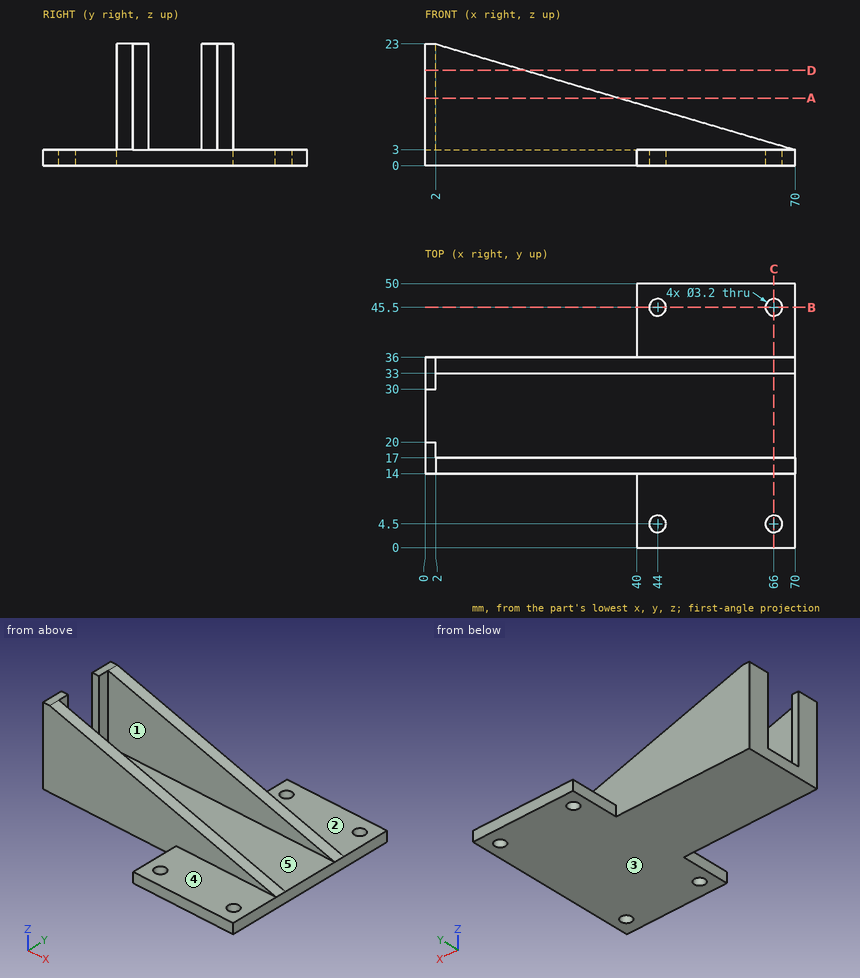
Input: dimensioned drawing with shaded views. Units: mm. Origin: part minimum x, y, z. A direction names the side the tool comes from. Coordinates: 2 decimals unless noted, no trailing zeros. Write each loop counter-clockwise with the first axis right and the second up, starting at its lowest first coordinate (ties: lowest second). Pieces come first, ordered by that corner, then holes. Notation, with made-up numbers: M 87,33.5 L 118,33.5 A24 cw 118,55.5 Z; hole C 87,83 d1. An arc over 180 degrees is marked long. Use one line per item in the form item = value.
Q1. Section D-D (z = 18). Return loops of the section in (x, y), plus the area to 3 significant figures.
Answer below:
outline = M 0,14 L 19,14 L 19,17 L 2,17 L 2,20 L 0,20 Z; M 0,30 L 2,30 L 2,33 L 19,33 L 19,36 L 0,36 Z
area = 126 mm²
Q2. Section C-C (x = 66). Return loops of the section in (y, z).
Answer below:
outline = M 0,0 L 2.9,0 L 2.9,3 L 0,3 Z; M 6.1,0 L 43.9,0 L 43.9,3 L 36,3 L 36,4.18 L 33,4.18 L 33,3 L 17,3 L 17,4.18 L 14,4.18 L 14,3 L 6.1,3 Z; M 47.1,0 L 50,0 L 50,3 L 47.1,3 Z
Q3. Draft query along Y for the marked faces 4 and 5. Return one class per face: released by +Y, released by -Y, zero draft, split by the parting line, or undercut.
Answer below:
face_4 = zero draft
face_5 = undercut
Q4. Section A-A (z = 12.75). Return loops of the section in (x, y), plus the area to 3 significant figures.
Answer below:
outline = M 0,14 L 36.85,14 L 36.85,17 L 2,17 L 2,20 L 0,20 Z; M 0,30 L 2,30 L 2,33 L 36.85,33 L 36.85,36 L 0,36 Z
area = 233 mm²
Q5. Set-up query: the marked faces 1, 2 and 3. Return all of +Z, -Z, +X, -X, +Y, -Y with unobstructed straight access to the full face (end or side cutting, diameter ignored); none if empty.
Answer below:
face_1 = +Z, +X
face_2 = +Z, +X, -X, +Y
face_3 = -Z, +X, -X, +Y, -Y
Q6. Material intervals for probe 1 along Y at (x, z) = (66, 1); probe 2 along Y at (x, z) = (11.5, 18.75); probe 3 along Z at (x, y) = (64, 31.5), sorted ascending. Write a range as from..to.
Answer below:
probe_1 = 0..2.9, 6.1..43.9, 47.1..50
probe_2 = 14..17, 33..36
probe_3 = 0..3
Q7. Section B-B (y = 45.5). Return loops of the section in (x, z).
Answer below:
outline = M 40,0 L 42.4,0 L 42.4,3 L 40,3 Z; M 45.6,0 L 64.4,0 L 64.4,3 L 45.6,3 Z; M 67.6,0 L 70,0 L 70,3 L 67.6,3 Z
Q8. First-contact query: pin 1 (12 mm diameter, centred on x = 34.5, z = 6, fed in from -Y); pin 2 (3.5 mm diameter, centred on y = 42, z = 1, fed in from -X); pin 3 (1 mm diameter, centred on x = 47, y = 12, fed in from -Z); pin 4 (3 mm diameter, centred on x = 44, y = 4.5, fed in from -Z). Flat tips, straight axial feed; report the tip coordinate or a pass-through.
Answer below:
pin_1 = 14
pin_2 = 40
pin_3 = 0
pin_4 = through
